```python
from build123d import *

# Parameters (mm, degrees)
CROQUIS1_W              = 19.5
CROQUIS1_H              = 15.4
CROQUIS1_R              = 1
SALIENTE_EXTRUIR1_DEPTH = 1
CROQUIS2_R              = 6
SALIENTE_EXTRUIR2_DEPTH = 10
CROQUIS3_W              = 2.54
CROQUIS3_H              = 7.62
SALIENTE_EXTRUIR3_DEPTH = 2.54
CROQUIS4_W              = 1
CROQUIS4_H              = 1
SALIENTE_EXTRUIR4_DEPTH = 2.54
CROQUIS6_W              = 1
CROQUIS6_H              = 1
SALIENTE_EXTRUIR5_DEPTH = 5.08
REDONDEO2_R             = 1
REDONDEO3_R             = 1
REDONDEO4_R             = 1
REDONDEO5_R             = 0.5
REDONDEO6_R             = 0.5
REDONDEO7_R             = 0.5


with BuildPart() as part:
    # Croquis1 → Saliente-Extruir1 (new body)
    with BuildSketch(Plane.XY):
        with Locations((-9.362960818, 4.807039504)):
            Rectangle(CROQUIS1_W, CROQUIS1_H)
        with Locations((-1.112960818, -1.392960496)):
            Circle(CROQUIS1_R, mode=Mode.SUBTRACT)
        with Locations((-1.112960818, 11.107039504)):
            Circle(CROQUIS1_R, mode=Mode.SUBTRACT)
    extrude(amount=SALIENTE_EXTRUIR1_DEPTH)

    # Croquis2 → Saliente-Extruir2 (add)
    with BuildSketch(Plane.XY.offset(1)):
        with Locations((-9.362960818, 4.807039504)):
            Circle(CROQUIS2_R)
    extrude(amount=SALIENTE_EXTRUIR2_DEPTH)

    # Croquis3 → Saliente-Extruir3 (add)
    with BuildSketch(Plane.XY.offset(1)):
        with Locations((-17.75568674, 4.807039504)):
            Rectangle(CROQUIS3_W, CROQUIS3_H)
    extrude(amount=SALIENTE_EXTRUIR3_DEPTH)

    # Croquis4 → Saliente-Extruir4 (add)
    with BuildSketch(Plane.XY.offset(3.54)):
        with Locations((-17.786846734, 7.347039504)):
            Rectangle(CROQUIS4_W, CROQUIS4_H)
        with Locations((-17.786846734, 4.807039504)):
            Rectangle(CROQUIS4_W, CROQUIS4_H)
        with Locations((-17.786846734, 2.267039504)):
            Rectangle(CROQUIS4_W, CROQUIS4_H)
    extrude(amount=SALIENTE_EXTRUIR4_DEPTH)

    # Croquis6 → Saliente-Extruir5 (add)
    with BuildSketch(Plane.ZY.offset(18.286846734)):
        with Locations((5.58, 4.807039504)):
            Rectangle(CROQUIS6_W, CROQUIS6_H)
        with Locations((5.58, 2.267039504)):
            Rectangle(CROQUIS6_W, CROQUIS6_H)
        with Locations((5.58, 7.347039504)):
            Rectangle(CROQUIS6_W, CROQUIS6_H)
    extrude(amount=SALIENTE_EXTRUIR5_DEPTH)

    # Redondeo2
    redondeo2_edges = [part.edges().sort_by_distance(p)[0] for p in [
        (-17.286846734, 2.267039504, 6.08),
    ]]
    fillet(redondeo2_edges, radius=REDONDEO2_R)

    # Redondeo3
    redondeo3_edges = [part.edges().sort_by_distance(p)[0] for p in [
        (-17.286846734, 4.807039504, 6.08),
    ]]
    fillet(redondeo3_edges, radius=REDONDEO3_R)

    # Redondeo4
    redondeo4_edges = [part.edges().sort_by_distance(p)[0] for p in [
        (-17.286846734, 7.347039504, 6.08),
    ]]
    fillet(redondeo4_edges, radius=REDONDEO4_R)

    # Redondeo5
    redondeo5_edges = [part.edges().sort_by_distance(p)[0] for p in [
        (-18.286846734, 2.267039504, 5.08),
    ]]
    fillet(redondeo5_edges, radius=REDONDEO5_R)

    # Redondeo6
    redondeo6_edges = [part.edges().sort_by_distance(p)[0] for p in [
        (-18.286846734, 4.807039504, 5.08),
    ]]
    fillet(redondeo6_edges, radius=REDONDEO6_R)

    # Redondeo7
    redondeo7_edges = [part.edges().sort_by_distance(p)[0] for p in [
        (-18.286846734, 7.347039504, 5.08),
    ]]
    fillet(redondeo7_edges, radius=REDONDEO7_R)


solid = part.part
```
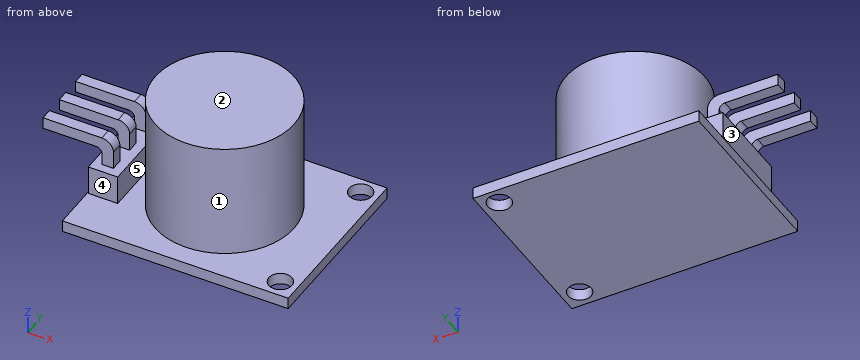
Build history of the part. All positions in model axes, mm. Face numbers are marked on the shaded views. A direction names the side the tool comes from. Round coordinates to 2 decimals unless told otherwise and drop trailing zeros. Write each loop counter-clockwise with the first axis right and the second up, starting at its lowest first coordinate (ties: lowest second). Pieces come first, ordered by that corner, then holes.
1) 3-axis set-ups, long thin cutter, end or side, ignore diameter. For the marked faces 1 and 2: which of +Z, -Z, +X, -X, +Y, -Y reach the whole face in a straight line?
2) Band-saw the part on A-A, the plane x = -21.5. List the corners of the cut face in (y, z).
3) Band-saw the part on C-C, the plane x = -17. List the corners of the cut face in (y, z).
4) Drill centre lines: probe 1 along Y at (x, z) = (-19.5, 5.25); probe 2 along Z at (x, y) = (-18.75, 5); probe 3 along Z at (x, y) = (-11, 10.75). Where is each one in solid material? Low to high.
5) Pin check, flat tips, straight feed: pin 1 (1.3 mm diameter, centred on x = -19, z = 5, fed in from +Y); pin 2 (0.8 mm diameter, centred on y = 7.5, z = 0.5, fed in from -X); pin 3 (3 mm diameter, centred on x = -1.11, y = 11.11, fed in from +Z). Stop position of each tip, or through.
6) Band-saw the part on B-B, the plane y = 11.75. List the corners of the cut face in (x, z), and give its area (3 significant figures).
7) Band-saw the part on D-D, the plane y = 2.5. List the corners of the cut face in (x, z).
8) Mould opens along X. For the marked faces 3, 4 and 5 say: +X half, -X half, draft (parallel to the pull), parting line (faces both ways), or undercut.
Ans:
1. face 1: +Z
1. face 2: +Z, +X, -X, +Y, -Y
2. outline: (1.77, 5.08) - (2.77, 5.08) - (2.77, 6.08) - (1.77, 6.08) - close; (4.31, 5.08) - (5.31, 5.08) - (5.31, 6.08) - (4.31, 6.08) - close; (6.85, 5.08) - (7.85, 5.08) - (7.85, 6.08) - (6.85, 6.08) - close
3. outline: (-2.89, 0) - (12.51, 0) - (12.51, 1) - (8.62, 1) - (8.62, 3.54) - (1, 3.54) - (1, 1) - (-2.89, 1) - close
4. probe 1: y = 1.77 to 2.77, 4.31 to 5.31, 6.85 to 7.85
4. probe 2: z = 0 to 3.54, 5.08 to 6.08
4. probe 3: z = 0 to 1
5. pin 1: stops at y = 7.85
5. pin 2: stops at x = -19.11
5. pin 3: stops at z = 1
6. outline: (-19.11, 0) - (-1.88, 0) - (-1.88, 1) - (-19.11, 1) - close; (-0.35, 0) - (0.39, 0) - (0.39, 1) - (-0.35, 1) - close
6. area: 18.0 mm2
7. outline: (-23.37, 5.08) - (-18.79, 5.08) arc R0.5 cw to (-18.29, 4.58) - (-18.29, 3.54) - (-19.03, 3.54) - (-19.03, 1) - (-19.11, 1) - (-19.11, 0) - (0.39, 0) - (0.39, 1) - (-3.82, 1) - (-3.82, 11) - (-14.9, 11) - (-14.9, 1) - (-16.49, 1) - (-16.49, 3.54) - (-17.29, 3.54) - (-17.29, 5.08) arc R1 ccw to (-18.29, 6.08) - (-23.37, 6.08) - close
8. face 3: -X half
8. face 4: draft
8. face 5: undercut
